Can you work these out from the model? Positions are in its coordinate system, mm. Face numbers are marked on the shaded views. Give positions to 0.01 mm unless a question says otherwise; leave off trailing zeros. Write each loop counter-clockwise with the first axis right and the second up, starting at its lowest first coordinate (ties: lowest second). Pieces come first, ordered by that corner, then holes. Notation, with made-up numbers: M 88.5,-27 L 122.5,-27 A25 cw 122.5,8 Z; hole C 83,41 d2. An arc over 180 degrees is marked long. Write each question's results on one line, items separated by ' | '.
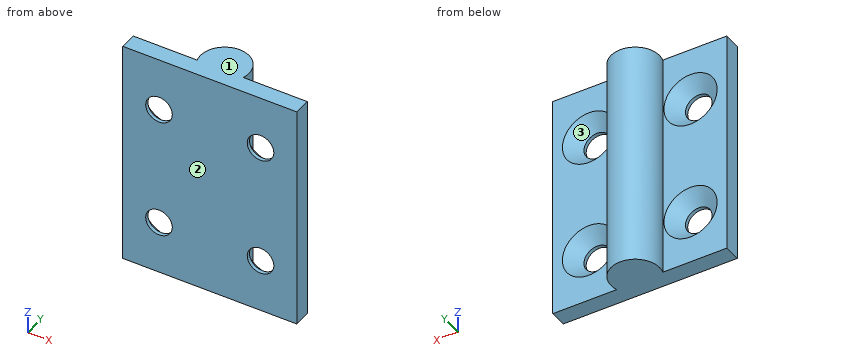
from build123d import *

# Parameters (mm, degrees)
SKETCH1_R           = 5
BOSS_EXTRUDE1_DEPTH = 23.5
HOLE1_AT_2_COUNT    = 2
HOLE1_AT_2_PITCH    = 25


with BuildPart() as part:
    # Sketch1 → Boss-Extrude1 (new, symmetric)
    with BuildSketch(Plane.XY):
        with BuildLine():
            Line((-18, -5), (0, -5))
            ThreePointArc((0, -5), (-2.958039892, -4.031128874), (-4.769696007, -1.5))
            Line((-4.769696007, -1.5), (-18, -1.5))
            Line((-18, -1.5), (-18, -5))
        make_face()
        Circle(SKETCH1_R)
    boss_extrude1 = extrude(amount=BOSS_EXTRUDE1_DEPTH, both=True)

    # Sketch5 → Hole1 (revolve, cut)
    with BuildSketch(Plane(origin=(-10.5, -1.5, -12.5), x_dir=(0, 0, 1), z_dir=(1, 0, 0))):
        Polygon((0, 0), (0, 5.152366702), (2.75, 3.5), (2.75, 2.75), (5.5, 0), align=None)
    hole1 = revolve(axis=Axis((-10.5, 12.808894879, -12.5), (0, -1, 0)), mode=Mode.SUBTRACT)

    # Hole1 at 2: Hole1 ×2
    with Locations(*[(0, 0, i * HOLE1_AT_2_PITCH) for i in range(1, HOLE1_AT_2_COUNT)]):
        add(hole1, mode=Mode.SUBTRACT)

    # Mirror1: Boss-Extrude1 across plane
    add(boss_extrude1.mirror(Plane(origin=(0, 0, 0), x_dir=(0, 0, 1), z_dir=(1, 0, 0))))

    # Mirror2: Hole1 across plane
    add(hole1.mirror(Plane(origin=(0, 0, 0), x_dir=(0, 0, 1), z_dir=(1, 0, 0))), mode=Mode.SUBTRACT)

    # Mirror2 copy 1 sketch → Mirror2 copy 1 (revolve, cut)
    with BuildSketch(Plane(origin=(10.5, -1.5, 12.5), x_dir=(0, 0, 1), z_dir=(-1, 0, 0))):
        Polygon((0, 0), (0, -5.152366702), (2.75, -3.5), (2.75, -2.75), (5.5, 0), align=None)
    revolve(axis=Axis((10.5, 12.808894879, 12.5), (0, 1, 0)), mode=Mode.SUBTRACT)


solid = part.part
Item 1: I'm going to push flat-ended pins straight in: pin 1 (5 mm diameter, centred on x = -10.5, z = -12.5, fed in from -Y); pin 2 (10.5 mm diameter, centred on x = -12, z = -5.5, fed in from +Y); pin 3 (2 mm diameter, centred on x = 8, z = -13, fed in from +Y); pin 4 (1.5 mm diameter, centred on x = 2.5, z = 14.5, fed in from +Y). Where does each tip first touch, or does it pass through?
Geometry says:
pin 1: passes through | pin 2: stops at y = -1.5 | pin 3: stops at y = -3.45 | pin 4: stops at y = 4.68
Item 2: Thinking about a two-plate mould opening in Z: for the marked faces 1, 2 and 3, which applies, +Z half, -Z half, draft (parallel to the pull), parting line (faces both ways), or undercut?
Geometry says:
face 1: +Z half | face 2: draft | face 3: undercut
Item 3: If I drill on line 1 (X direction, y = -4.45, z = 12.5); line 2 (Z direction, x = -10.5, y = -4.6); line 3 (X direction, y = -4, z = -12), over which ranges is the centre line in solid material (lowest first)? Write a range as from..to.
Geometry says:
line 1: x = -18..-13.25, -7.75..7.75, 13.25..18 | line 2: z = -23.5..-15.25, -9.75..9.75, 15.25..23.5 | line 3: x = -18..-13.46, -7.54..7.54, 13.46..18
Item 4: I want a section at D-D, the plane z = -2.5. Please give me the cut outline in (x, y), and give its area (3 significant figures).
Geometry says:
outline: M -18,-5 L 18,-5 L 18,-1.5 L 4.77,-1.5 A5 ccw long -4.77,-1.5 L -18,-1.5 Z | area: 180 mm2
Item 5: I want a section at A-A, the plane z = -12.5. Please give me the cut outline in (x, y).
Geometry says:
outline: M -18,-5 L -13.25,-5 L -13.25,-4.25 L -16,-1.5 L -18,-1.5 Z; M -7.75,-5 L 7.75,-5 L 7.75,-4.25 L 5,-1.5 L 4.77,-1.5 A5 ccw long -4.77,-1.5 L -5,-1.5 L -7.75,-4.25 Z; M 13.25,-5 L 18,-5 L 18,-1.5 L 16,-1.5 L 13.25,-4.25 Z
Item 6: I want a section at B-B, the plane x = -10.5. Please give me the cut outline in (y, z), and give its area (3 significant figures).
Geometry says:
outline: M -5,-23.5 L -1.5,-23.5 L -1.5,-18 L -4.25,-15.25 L -5,-15.25 Z; M -5,-9.75 L -4.25,-9.75 L -1.5,-7 L -1.5,7 L -4.25,9.75 L -5,9.75 Z; M -5,15.25 L -4.25,15.25 L -1.5,18 L -1.5,23.5 L -5,23.5 Z | area: 111 mm2
Item 7: I want a section at C-C, the plane y = 0. Please give me the cut outline in (x, z).
Geometry says:
outline: M -5,-23.5 L 5,-23.5 L 5,23.5 L -5,23.5 Z
